Autodesk Inventor part; units mm, degrees
ref_plane "YZ Plane" through (0, 0, 0) normal (1, 0, 0) x (0, 1, 0)
ref_plane "XZ Plane" through (0, 0, 0) normal (0, 1, 0) x (-1, 0, 0)
ref_plane "XY Plane" through (0, 0, 0) normal (0, 0, 1) x (1, 0, 0)
sketch "Sketch1" plane through (0, 0, 0) normal (1, 0, 0) x (0, 1, 0)
  circle A0 centre (0, 0) radius 62.5
  dimension "d0" = 125
extrude "Extrusion1" add sketch "Sketch1" along normal blind 36.5
fillet "Fillet1" radius 5 2 edges at (36.5, -62.5, 0) (0, -62.5, 0)
sketch "Sketch2" plane through (36.5, 0, 0) normal (1, 0, 0) x (0, 0, -1)
  circle A0 centre (0, 0) radius 62.5
hole "Hole1" at (36.5, 0, 0) direction (-1, 0, 0) diameter 20 end through all
sketch "Sketch3" plane through (36.5, 0, 0) normal (1, 0, 0) x (0, 0, -1)
  circle A0 centre (0, 0) radius 25
  dimension "d11" = 50
extrude "Extrusion2" cut sketch "Sketch3" against normal blind 8.5
sketch "Sketch4" plane through (28, 0, 0) normal (1, 0, 0) x (0, 0, -1)
  line L0 (-7, -3) -> (-13, -3)
  line L1 (-13, -3) -> (-13, 3)
  line L2 (-13, 3) -> (-7, 3)
  line L3 (-7, 3) -> (-7, -3)
  circle A0 centre (0, 0) radius 10
  line L4 (-7, -3) -> (-13, 3) construction
  line L5 (-13, -3) -> (-7, 3) construction
  point P0 (-10, 0)
  dimension "d14" = 6
  dimension "d15" = 6
extrude "Extrusion3" cut sketch "Sketch4" against normal blind 28 contours L0 A0 L2 L3 | L0 L1 L2 A0 picked at (-7.9828, 0.338)
properties part number "100mm Traction Wheel StandIn" material "Rubber"
CAD build for the part. Positions are in the model's coordinates, mm. A direction names the side the tool comes from. Coordinates: 2 decimals unless noted, no trailing zeros. Loops run counter-clockwise (first coordinate to the right, second up) from the corner with the lowest first, then second, coordinate; pieces in that order, holes last. Notation, with made-up numbers: (-27.5, -31) - (2.5, -31) arc R7 ccw to (2.5, -18) - close; hole circle Ø8 at (76.25, -3.5). An arc over 180 degrees is marked (long way). Use CSV: the item, a comma, the result in double quotes. Start each with the question number.
Q1. Cut at B-B, the plane z = 0. List the corners of the cut face in (x, y).
Q2. Cut at A-A, the plane y = 0. List the corners of the cut face in (x, z), then the cut area to 3 significant figures.
Q3. Probe probe 1 along Z at (x, y) = (12, 0); probe 2 along X at (y, z) = (-7.5, 22); probe 3 along Z at (x, y) = (29.5, 23). List the from-to ranges inside material, lowest first. Write a range as from..to.
Q4. Cut at C-C, the plane x = 19.5. List the corners of the cut face in (y, z).
Q5. Drop flat-ended pins along their axis: P1, Ø12, axis at x = 21.5, y = -38.5, coming from the -Z side; P2, Ø6.5, axis at x = 7, y = -0.5, coming from the -Z side; P3, Ø1, axis at x = 20, z = 10.5, coming from the +Y side. Give the stop position or say it passes through.
Q6. Two-plate mould, pull along Y, no slides. Class faces 4 (the flat face through (0, 12, 1)), 5 (the cylindrical face through (18.06, -62.44, -2.75)), 6 (the flat face through (14, 0, 13)): +Y half, -Y half, draft (parallel to the pull), parting line (faces both ways), or undercut.
Q7. 3-axis set-ups, long thin cutter, end or side, ignore diameter. For faces 1 (the flat face through (36.5, 12, -25)), 2 (the flat face through (14, -3, 11)), 3 (the flat face through (28, 0, -11)): which of +Z, -Z, +X, -X, +Y, -Y reach the whole face in a straight line?
Here are the results:
1,outline,"(0, -57.5) arc R5 ccw to (5, -62.5) - (31.5, -62.5) arc R5 ccw to (36.5, -57.5) - (36.5, -25) - (28, -25) - (28, -10) - (0, -10) - close; (0, 10) - (28, 10) - (28, 25) - (36.5, 25) - (36.5, 57.5) arc R5 ccw to (31.5, 62.5) - (5, 62.5) arc R5 ccw to (0, 57.5) - close"
2,outline,"(0, -57.5) arc R5 ccw to (5, -62.5) - (31.5, -62.5) arc R5 ccw to (36.5, -57.5) - (36.5, -25) - (28, -25) - (28, -10) - (0, -10) - close; (0, 13) - (28, 13) - (28, 25) - (36.5, 25) - (36.5, 57.5) arc R5 ccw to (31.5, 62.5) - (5, 62.5) arc R5 ccw to (0, 57.5) - close"
2,area,"3,470 mm2"
3,probe 1,"-62.5..-10, 13..62.5"
3,probe 2,"0..28"
3,probe 3,"-58.11..-9.8, 9.8..58.11"
4,outline,"circle Ø125 at (0, 0); hole (-3, 9.54) arc R10 ccw (long way) to (3, 9.54) - (3, 13) - (-3, 13) - close"
5,P1,"z = -53.39"
5,P2,"z = -62.5"
5,P3,"y = 61.69"
6,face 4,"draft"
6,face 5,"parting line"
6,face 6,"undercut"
7,face 1,"+Z, -Z, +X, +Y, -Y"
7,face 2,"+X, -X"
7,face 3,"+X"
